Could you check a few things on this model? Use its own coordinates, in mm. A direction names the side the tool comes from. Coordinates: 2 decimals unless noted, no trailing zeros. Write each loop counter-clockwise with the first axis right and the second up, starting at its lowest first coordinate (ties: lowest second). Pieces come first, ordered by that corner, then holes.
Item 1: I want a section at B-B on z = 17.5. Please give me the cut outline in (x, y), then the cut area to 3 significant figures.
Item 2: I want a section at A-A on z = 0. Please give me the cut outline in (x, y), then the cut area to 3 significant figures.
Item 3: Thinking about a two-plate mould opening in Z: for faces 1 (the flat face through (41, 1, 1)), 2 (the flat face through (37.76, 1, -19)), 3 (the flat face through (-1, 1, 32.385)), which applies, +Z half, -Z half, draft (parallel to the pull), parting line (faces both ways), or undercut?
Item 4: Which directions (+Z, -Z, +X, -X, +Y, -Y) give clear straight access to the entire face, cutting with the end or side of a thin tool? Please do faces 4 (the flat face through (-40, 1, 20)), 5 (the cylindrical face through (39.83, 1.51, -0.65)), 6 (the flat face through (40, 1, -5)), 7 (the flat face through (40, 1, 5)).
Item 5: I want a section at C-C on z = -12. Please give me the cut outline in (x, y), then the cut area to 3 significant figures.
Item 6: For P1, Ø4, axis at x = -40.5, z = -21, coming from the +Y side; P2, Ø0.5, axis at x = -39.5, y = 0.5, coming from the -Z side; P3, Ø0.8, axis at x = -39.5, y = 0.5, coming from the +Z side, each with a flat end and sliding along its axis, tell me the tip position at first contact or that it passes through.
Item 7: If I drill on probe 1 along X at (y, z) = (0.3, 0); probe 2 along X at (y, z) = (1.8, 0); probe 3 along X at (y, z) = (0.3, 6), over which ranges is the centre line in solid material (lowest first)?
from build123d import *

# Parameters (mm, degrees)
SKETCH1_W           = 75.52
SKETCH1_H           = 64.77
BOSS_EXTRUDE1_DEPTH = 2
BOSS_EXTRUDE2_DEPTH = 2
SKETCH3_W           = 10
SKETCH3_H           = 1
BOSS_EXTRUDE3_DEPTH = 5
SKETCH7_R           = 1.5
CUT_EXTRUDE2_DEPTH  = 2
SKETCH9_R           = 3
SKETCH9_R_2         = 1.5
CUT_EXTRUDE4_DEPTH  = 1
FILLET1_R           = 1


with BuildPart() as part:
    # Sketch1 → Boss-Extrude1 (new body)
    with BuildSketch(Plane(origin=(0, 0, 0), x_dir=(1, 0, 0), z_dir=(0, 1, 0))):
        Rectangle(SKETCH1_W, SKETCH1_H)
    extrude(amount=BOSS_EXTRUDE1_DEPTH)

    # Sketch2 → Boss-Extrude2 (add)
    with BuildSketch(Plane(origin=(0, 2, 0), x_dir=(1, 0, 0), z_dir=(0, 1, 0))):
        with BuildLine():
            Line((37.76, 5), (42.76, 5))
            ThreePointArc((42.76, 5), (47.76, 0), (42.76, -5))
            Line((42.76, -5), (37.76, -5))
            Line((37.76, -5), (37.76, 5))
        make_face()
    extrude(amount=-BOSS_EXTRUDE2_DEPTH)

    # Sketch3 → Boss-Extrude3 (add)
    with BuildSketch(Plane.ZY.offset(37.76)):
        with Locations((-20, 0.5)):
            Rectangle(SKETCH3_W, SKETCH3_H)
        with Locations((20, 0.5)):
            Rectangle(SKETCH3_W, SKETCH3_H)
    extrude(amount=BOSS_EXTRUDE3_DEPTH)

    # Sketch7 → Cut-Extrude2 (cut)
    with BuildSketch(Plane(origin=(0, 2, 0), x_dir=(1, 0, 0), z_dir=(0, 1, 0))):
        with Locations(Location((42.76, 0, 0), (0, 0, 270))):
            Circle(SKETCH7_R)
    extrude(amount=-CUT_EXTRUDE2_DEPTH, mode=Mode.SUBTRACT)

    # Sketch9 → Cut-Extrude4 (cut)
    with BuildSketch(Plane(origin=(0, 2, 0), x_dir=(1, 0, 0), z_dir=(0, 1, 0))):
        with Locations(Location((42.76, 0, 0), (0, 0, 270))):
            Circle(SKETCH9_R)
        with Locations(Location((42.76, 0, 0), (0, 0, 270))):
            Circle(SKETCH9_R_2, mode=Mode.SUBTRACT)
    extrude(amount=-CUT_EXTRUDE4_DEPTH, mode=Mode.SUBTRACT)

    # Fillet1
    fillet1_edges = [part.edges().sort_by_distance(p)[0] for p in [
        (-42.76, 0.5, -15),
        (-42.76, 0.5, -25),
        (-42.76, 0.5, 25),
        (-42.76, 0.5, 15),
    ]]
    fillet(fillet1_edges, radius=FILLET1_R)


solid = part.part
Response values:
1. outline: (-42.76, 0) - (37.76, 0) - (37.76, 2) - (-37.76, 2) - (-37.76, 1) - (-42.76, 1) - close
1. area: 156 mm2
2. outline: (-37.76, 0) - (41.26, 0) - (41.26, 1) - (39.76, 1) - (39.76, 2) - (-37.76, 2) - close; (44.26, 0) - (47.76, 0) - (47.76, 2) - (45.76, 2) - (45.76, 1) - (44.26, 1) - close
2. area: 162 mm2
3. face 1: undercut
3. face 2: draft
3. face 3: +Z half
4. face 4: +Z, -Z, -X, +Y
4. face 5: +Y
4. face 6: -Z, +X, +Y, -Y
4. face 7: +Z, +X, +Y, -Y
5. outline: (-37.76, 0) - (37.76, 0) - (37.76, 2) - (-37.76, 2) - close
5. area: 151 mm2
6. P1: stops at y = 1
6. P2: stops at z = -25
6. P3: stops at z = 25
7. probe 1: x = -37.76 to 41.26, 44.26 to 47.76
7. probe 2: x = -37.76 to 39.76, 45.76 to 47.76
7. probe 3: x = -37.76 to 37.76
